Autodesk Inventor part; units mm, degrees
ref_plane "YZ Plane" through (0, 0, 0) normal (1, 0, 0) x (0, 1, 0)
ref_plane "XZ Plane" through (0, 0, 0) normal (0, 1, 0) x (-1, 0, 0)
ref_plane "XY Plane" through (0, 0, 0) normal (0, 0, 1) x (1, 0, 0)
sketch "Sketch1" plane through (0, 0, 0) normal (0, 1, 0) x (-1, 0, 0)
  line L0 (42, 0) -> (-42, 0)
  line L1 (0, -19.2) -> (0, 3.2)
  line L2 (30, -16) -> (-30, -16)
  line L3 (-30, -16) -> (-30, 0)
  line L4 (-30, 0) -> (30, 0)
  line L5 (30, 0) -> (30, -16)
  point P0 (0, 0)
  dimension "d0" = 16
  dimension "d1" = 60
extrude "Extrusion1" add sketch "Sketch1" along normal blind 6
sketch "Sketch2" plane through (0, 6, 0) normal (0, 1, 0) x (1, 0, 0)
  line L0 (30, 16) -> (-30, 16)
  line L1 (-30, 16) -> (-30, 0)
  line L2 (-30, 0) -> (30, 0)
  line L3 (30, 0) -> (30, 16)
  line L4 (0, 19.2) -> (0, -3.2)
  line L5 (-42, 0) -> (42, 0)
  point P0 (0, 0)
  point P1 (-23, 8)
  point P2 (23, 8)
  dimension "d4" = 7
  dimension "d5" = 7
  dimension "d6" = 8
  dimension "d7" = 8
hole "Hole1" at (23, 6, -8) at (-23, 6, -8) direction (0, -1, 0) diameter 7 end through all
sketch "Sketch3" plane through (0, 6, 0) normal (0, 1, 0) x (1, 0, 0)
  circle A0 centre (23, 8) radius 3.5
  circle A1 centre (-23, 8) radius 3.5
  line L0 (30, 16) -> (-30, 16)
  line L1 (-30, 16) -> (-30, 0)
  line L2 (-30, 0) -> (30, 0)
  line L3 (30, 0) -> (30, 16)
  line L4 (0, 19.2) -> (0, -3.2)
  line L5 (-23, 8) -> (23, 8) construction
  point P0 (0, 0)
  point P1 (-14.5, 8)
  point P2 (14.5, 8)
  dimension "d15" = 8.5
  dimension "d16" = 8.5
hole "Hole2" at (-14.5, 6, -8) at (14.5, 6, -8) direction (0, -1, 0) diameter 1.5 end through all
fillet "Fillet1" radius 7 4 edges at (30, 3, -16) (30, 3, 0) (-30, 3, -16) (-30, 3, 0)
fillet "Fillet2" radius 1 16 edges at (0, 0, 0) (-27.9497, 0, -2.0503) (-30, 0, -8) (-27.9497, 0, -13.9497) (0, 0, -16) (27.9497, 0, -13.9497) (30, 0, -8) (27.9497, 0, -2.0503) (27.9497, 6, -2.0503) (30, 6, -8) (27.9497, 6, -13.9497) (0, 6, -16) (-27.9497, 6, -13.9497) (-30, 6, -8) (-27.9497, 6, -2.0503) (0, 6, 0)
properties part number "femur_v3"
Input: part model. Units: mm. Frame: model coordinates. Coordinates: 2 decimals unless noted, no trailing zeros. Loops run counter-clockwise (first coordinate to the right, second up) from the corner with the lowest first, then second, coordinate; pieces in that order, holes last. Notation, with made-up numbers: (72, 4) -> (98, 4) arc R25 cw to (98, 17) -> close; hole circle Ø5 at (24.5, 42). An arc over 180 degrees is marked (long way). Write item = value, one per line. Start each with the question number.
Item 1: Material intervals for line 1 (X direction, y = 4.3, z = -8); line 2 (Z direction, x = -14.5, y = 1.65); line 3 (X direction, y = 3.8, z = -6.5), sorted ascending.
Item 2: Cut plane A-A, the plane x = 14.5. Return loops of the section in (y, z), plus the area to 3 significant figures.
Item 3: Cut plane B-B, the plane y = 1.55. Return loops of the section in (x, z), plus the area to 3 significant figures.
Item 4: Mould query, pull axis X, two halves, no side actions, for faces 1 (the face through (13.99, 2.96, -8.55)), 2 (the face through (0, 0, -8)), 3 (the face through (29.699, 5.715, -8.014)). Classes: pulls with the +X half, pulls with the -X half, needs draft (parallel to the pull), parting line crosses it, or undercut.
Item 5: Cut plane D-D, the plane z = -5.75. Count the separate pieces of the cut face and the enclosed holes in it, plus the area to 3 significant figures.
Item 6: Cut plane C-C, the plane z = -8. Return loops of the section in (x, y), plus the area to 3 significant figures.
Ans:
q1.line_1 = -30 to -26.5, -19.5 to -15.25, -13.75 to 13.75, 15.25 to 19.5, 26.5 to 30
q1.line_2 = -16 to -8.75, -7.25 to 0
q1.line_3 = -29.98 to -26.16, -19.84 to 19.84, 26.16 to 29.98
q2.outline = (0, -15) arc R1 ccw to (1, -16) -> (5, -16) arc R1 ccw to (6, -15) -> (6, -8.75) -> (0, -8.75) -> close; (0, -7.25) -> (6, -7.25) -> (6, -1) arc R1 ccw to (5, 0) -> (1, 0) arc R1 ccw to (0, -1) -> close
q2.area = 86.1 mm²
q3.outline = (-30, -9) arc R7 ccw to (-23, -16) -> (23, -16) arc R7 ccw to (30, -9) -> (30, -7) arc R7 ccw to (23, 0) -> (-23, 0) arc R7 ccw to (-30, -7) -> close; hole circle Ø7 at (-23, -8); hole circle Ø1.5 at (-14.5, -8); hole circle Ø1.5 at (14.5, -8); hole circle Ø7 at (23, -8)
q3.area = 837 mm²
q4.face_1 = undercut
q4.face_2 = needs draft
q4.face_3 = pulls with the +X half
q5.separate_pieces = 3
q5.enclosed_holes = 0
q5.area = 293 mm²
q6.outline = (-30, 1) arc R1 ccw to (-29, 0) -> (-26.5, 0) -> (-26.5, 6) -> (-29, 6) arc R1 ccw to (-30, 5) -> close; (-19.5, 0) -> (-15.25, 0) -> (-15.25, 6) -> (-19.5, 6) -> close; (-13.75, 0) -> (13.75, 0) -> (13.75, 6) -> (-13.75, 6) -> close; (15.25, 0) -> (19.5, 0) -> (19.5, 6) -> (15.25, 6) -> close; (26.5, 0) -> (29, 0) arc R1 ccw to (30, 1) -> (30, 5) arc R1 ccw to (29, 6) -> (26.5, 6) -> close
q6.area = 257 mm²
